Geometry: see drawing. Coordinates: mm, zero at the bounding-box minimum. Give positions to 0.01 mm unless a question says otherwise; leave off trailing zeros. Write each loop counter-clockwise with the first axis right and the second up, starting at its lowest first coordinate (ties: lowest second). Pieces come first, ordered by that corner, then holes. Notation, with made-up numbers: (-21.5, 69) -> (31.5, 69) arc R29 ccw to (31.5, 90) -> close; hole circle Ø9 at (-2, 53). An arc over 180 degrees is marked (long way). Answer as a JSON object with one key per item and string values. Group by question number.
Item 1: First-contact query: pin 1 Ø1.5 at (y, z) = (1, 17) entering from +X. Flat tip, straight axial feed; report the tip coordinate or a pass-through.
Item 2: Section query A-A on z = 15. Return the cut outline in (x, y), plus the area to 3 significant figures.
Item 3: Section query C-C on y = 1.05. Return the cut outline in (x, z), plus the area to 3 significant figures.
Item 4: Section query B-B on x = 97. Return the cut outline in (y, z).
Item 5: Section query D-D on z = 25. Return the cut outline in (x, y), plus the area to 3 significant figures.
Item 6: Ray query, probe 1 along Z at (x, y) = (97, 1.5); probe 2 along X at (y, z) = (2, 22); probe 3 along X at (y, z) = (2.5, 14.25). Return the intervals inside material, ascending. Write a range as from..to.
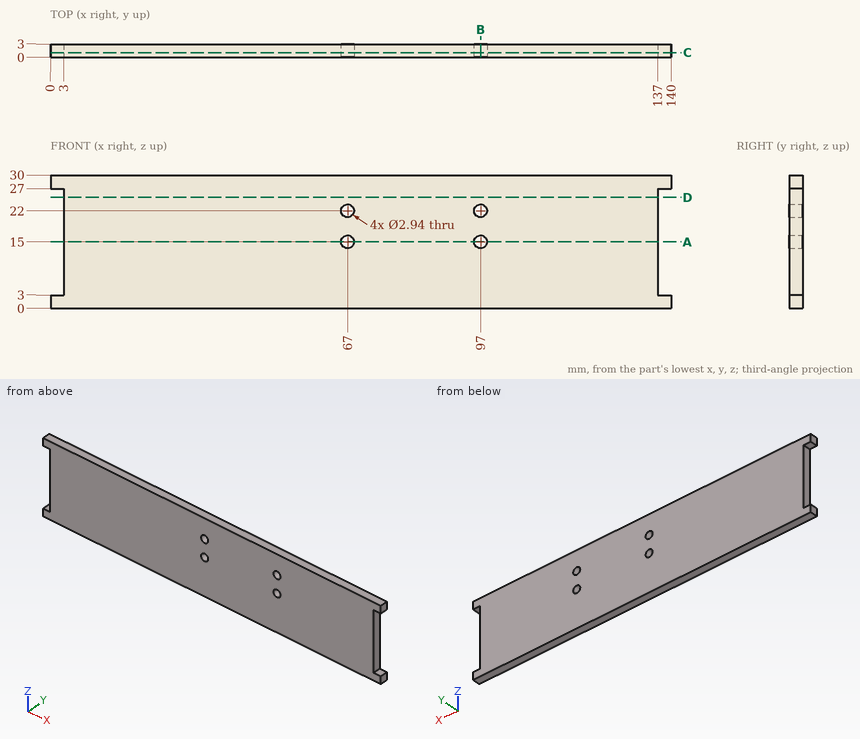
Worked answers:
{
 "1": {"pin 1": "x = 137"},
 "2": {"outline": "(3, 0) -> (65.53, 0) -> (65.53, 3) -> (3, 3) -> close; (68.47, 0) -> (95.53, 0) -> (95.53, 3) -> (68.47, 3) -> close; (98.47, 0) -> (137, 0) -> (137, 3) -> (98.47, 3) -> close", "area": "384 mm^2"},
 "3": {"outline": "(0, 0) -> (140, 0) -> (140, 3) -> (137, 3) -> (137, 27) -> (140, 27) -> (140, 30) -> (0, 30) -> (0, 27) -> (3, 27) -> (3, 3) -> (0, 3) -> close; hole circle Ø2.94 at (67, 15); hole circle Ø2.94 at (67, 22); hole circle Ø2.94 at (97, 15); hole circle Ø2.94 at (97, 22)", "area": "4,030 mm^2"},
 "4": {"outline": "(0, 0) -> (3, 0) -> (3, 13.53) -> (0, 13.53) -> close; (0, 16.47) -> (3, 16.47) -> (3, 20.53) -> (0, 20.53) -> close; (0, 23.47) -> (3, 23.47) -> (3, 30) -> (0, 30) -> close"},
 "5": {"outline": "(3, 0) -> (137, 0) -> (137, 3) -> (3, 3) -> close", "area": "402 mm^2"},
 "6": {"probe 1": "0..13.53, 16.47..20.53, 23.47..30", "probe 2": "3..65.53, 68.47..95.53, 98.47..137", "probe 3": "3..65.74, 68.26..95.74, 98.26..137"}
}
